Input: part model. Units: mm. Frame: model coordinates. Give positions to 0.01 mm unless a question says otherwise; leave off trailing zeros. Answer as a JSON object with one key per item and string values.
```python
from build123d import *

# Parameters (mm, degrees)
EXTRUDE_2_DEPTH     = 100
SKETCH_7_R          = 1.5
CUT_EXTRUDE_1_DEPTH = 100


with BuildPart() as part:
    # По траектории3: sweep along a path in Эскиз3
    with BuildLine(Plane(origin=(0, 0, 0), x_dir=(0, 0, -1), z_dir=(1, 0, 0))) as sweep_3_path:
        ThreePointArc((0, 3), (-25, 3.625391114), (-50, 3))
    # Эскиз1 → По траектории3 (sweep)
    with BuildSketch(Plane.XY):
        with BuildLine():
            Line((0, 0), (100, 0))
            Line((100, 0), (100, 3))
            ThreePointArc((100, 3), (50, 5.506281447), (0, 3))
            Line((0, 3), (0, 0))
        make_face()
    sweep(path=sweep_3_path.line)

    # Эскиз6 → Бобышка-Вытянуть2 (add)
    with BuildSketch(Plane.ZY):
        Polygon((0, 0), (49.700375235, 0.015), (50, 3), (0, 3), align=None)
    extrude(amount=-EXTRUDE_2_DEPTH)

    # Эскиз7 → Вырез-Вытянуть1 (cut)
    with BuildSketch(Plane(origin=(0, 0, 0), x_dir=(1, 0, 0), z_dir=(0, -0.9999999544557917, 0.00030180857279200576))):
        with Locations(Location((80, 34.700377498, 0), (0, 0, 270))):
            Circle(SKETCH_7_R)
        with Locations(Location((71.5, 15, 0), (0, 0, 270))):
            Circle(SKETCH_7_R)
        with Locations(Location((88.5, 15, 0), (0, 0, 270))):
            Circle(SKETCH_7_R)
    extrude(amount=-CUT_EXTRUDE_1_DEPTH, mode=Mode.SUBTRACT)


solid = part.part
```
Q1. Ray query, line 1 along X through (y, z) = (2.5, 15); line 2 along Z through (x, y) = (88.5, 2.85); line 3 along Z through (x, y) = (80, 1.3). Return the intervals inside material, ascending.
Evaluation:
{"line 1": "x = 0 to 70, 73 to 87, 90 to 100", "line 2": "z = 0 to 13.5, 16.5 to 49.98", "line 3": "z = 0 to 33.2, 36.2 to 49.83"}
Q2. Section A-A, the plane z = 15. Give the number of separate pieces and of enclosed holes in the cut face, then the cut area to 3 significant figures.
Evaluation:
{"separate pieces": "3", "enclosed holes": "0", "area": "489 mm2"}
Q3. Draft query along Z for faces 1 (the cylindrical face through (81.487, 2.583, 34.895)), 2 (the flat face through (100, 2, 25)), 3 (the flat face through (49, 2, 0)). Return one class per face: +Z half, -Z half, draft (parallel to the pull), parting line (faces both ways), or undercut.
Evaluation:
{"face 1": "undercut", "face 2": "draft", "face 3": "-Z half"}
Q4. Pin query (flat end, axial travel): pin 1 (1.5 mm diameter, centred on x = 77, z = 28, fed in from -Y); pin 2 (1.8 mm diameter, centred on x = 71.5, z = 15, fed in from -Y); pin 3 (4 mm diameter, centred on x = 80, z = 34.7, fed in from +Y). Return the tip coordinate at first contact, or that it passes through.
Evaluation:
{"pin 1": "stops at y = 0.01", "pin 2": "passes through", "pin 3": "stops at y = 5.26"}
